Autodesk Inventor part; units mm, degrees
ref_plane "YZ Plane" through (0, 0, 0) normal (1, 0, 0) x (0, 1, 0)
ref_plane "XZ Plane" through (0, 0, 0) normal (0, 1, 0) x (-1, 0, 0)
ref_plane "XY Plane" through (0, 0, 0) normal (0, 0, 1) x (1, 0, 0)
sketch "Sketch1" plane through (0, 0, 0) normal (0, 1, 0) x (-1, 0, 0)
  line L0 (-104, 150) -> (104, 150)
  line L1 (150, 104) -> (150, -104)
  line L2 (104, -150) -> (-104, -150)
  line L3 (-150, -104) -> (-150, 104)
  line L4 (-150, 150) -> (150, -150) construction
  line L5 (150, 150) -> (-150, -150) construction
  line L6 (-100, 100) -> (100, 100) construction
  line L7 (100, 100) -> (100, -100) construction
  line L8 (100, -100) -> (-100, -100) construction
  line L9 (-100, -100) -> (-100, 100) construction
  line L10 (-100, 100) -> (100, -100) construction
  line L11 (100, 100) -> (-100, -100) construction
  line L12 (-125, 125) -> (125, 125) construction
  line L13 (125, 125) -> (125, -125) construction
  line L14 (125, -125) -> (-125, -125) construction
  line L15 (-125, -125) -> (-125, 125) construction
  line L16 (-125, 125) -> (125, -125) construction
  line L17 (125, 125) -> (-125, -125) construction
  line L18 (-75, 75) -> (75, 75) construction
  line L19 (75, 75) -> (75, -75) construction
  line L20 (75, -75) -> (-75, -75) construction
  line L21 (-75, -75) -> (-75, 75) construction
  line L22 (-75, 75) -> (75, -75) construction
  line L23 (75, 75) -> (-75, -75) construction
  line L24 (-104, -104) -> (104, -104) construction
  line L25 (104, -104) -> (104, 104) construction
  line L26 (104, 104) -> (-104, 104) construction
  line L27 (-104, 104) -> (-104, -104) construction
  circle A0 centre (125, -125) radius 1.5
  circle A1 centre (75, -75) radius 1.5
  circle A2 centre (75, 75) radius 1.5
  circle A3 centre (125, 125) radius 1.5
  circle A4 centre (-75, 75) radius 1.5
  circle A5 centre (-125, 125) radius 1.5
  circle A6 centre (-75, -75) radius 1.5
  circle A7 centre (-125, -125) radius 1.5
  line L28 (17.5, -100) -> (-17.5, -100)
  line L29 (-17.5, -100) -> (-17.5, -104)
  line L30 (-17.5, -104) -> (17.5, -104)
  line L31 (17.5, -104) -> (17.5, -100)
  arc A8 (104, -150) -> (150, -104) centre (104, -104) ccw
  arc A9 (150, 104) -> (104, 150) centre (104, 104) ccw
  arc A10 (-150, -104) -> (-104, -150) centre (-104, -104) ccw
  arc A11 (-104, 150) -> (-150, 104) centre (-104, 104) ccw
  line L32 (87.5, -100) -> (52.5, -100)
  line L33 (52.5, -100) -> (52.5, -104)
  line L34 (52.5, -104) -> (87.5, -104)
  line L35 (87.5, -104) -> (87.5, -100)
  line L36 (-87.5, -100) -> (-52.5, -100)
  line L37 (-52.5, -100) -> (-52.5, -104)
  line L38 (-52.5, -104) -> (-87.5, -104)
  line L39 (-87.5, -104) -> (-87.5, -100)
  line L40 (52.5, -104) -> (17.5, -100) construction
  line L41 (-17.5, -100) -> (-52.5, -104) construction
  line L42 (100, 17.5) -> (100, -17.5)
  line L43 (104, -17.5) -> (104, 17.5)
  line L44 (104, 17.5) -> (100, 17.5)
  line L45 (100, 52.5) -> (104, 52.5)
  line L46 (100, 87.5) -> (100, 52.5)
  line L47 (104, 87.5) -> (100, 87.5)
  line L48 (104, 52.5) -> (104, 87.5)
  line L49 (104, 52.5) -> (100, 17.5) construction
  line L50 (100, -17.5) -> (104, -17.5)
  line L51 (100, -17.5) -> (104, -52.5) construction
  line L52 (100, -52.5) -> (104, -52.5)
  line L53 (104, -87.5) -> (100, -87.5)
  line L54 (104, -52.5) -> (104, -87.5)
  line L55 (100, -87.5) -> (100, -52.5)
  line L56 (-17.5, 100) -> (17.5, 100)
  line L57 (17.5, 104) -> (-17.5, 104)
  line L58 (-17.5, 104) -> (-17.5, 100)
  line L59 (-52.5, 100) -> (-52.5, 104)
  line L60 (-87.5, 100) -> (-52.5, 100)
  line L61 (-87.5, 104) -> (-87.5, 100)
  line L62 (-52.5, 104) -> (-87.5, 104)
  line L63 (-52.5, 104) -> (-17.5, 100) construction
  line L64 (17.5, 100) -> (17.5, 104)
  line L65 (17.5, 100) -> (52.5, 104) construction
  line L66 (52.5, 100) -> (52.5, 104)
  line L67 (87.5, 104) -> (87.5, 100)
  line L68 (52.5, 104) -> (87.5, 104)
  line L69 (87.5, 100) -> (52.5, 100)
  line L70 (-100, -17.5) -> (-100, 17.5)
  line L71 (-104, 17.5) -> (-104, -17.5)
  line L72 (-104, -17.5) -> (-100, -17.5)
  line L73 (-100, -52.5) -> (-104, -52.5)
  line L74 (-100, -87.5) -> (-100, -52.5)
  line L75 (-104, -87.5) -> (-100, -87.5)
  line L76 (-104, -52.5) -> (-104, -87.5)
  line L77 (-104, -52.5) -> (-100, -17.5) construction
  line L78 (-100, 17.5) -> (-104, 17.5)
  line L79 (-100, 17.5) -> (-104, 52.5) construction
  line L80 (-100, 52.5) -> (-104, 52.5)
  line L81 (-104, 87.5) -> (-100, 87.5)
  line L82 (-104, 52.5) -> (-104, 87.5)
  line L83 (-100, 87.5) -> (-100, 52.5)
  point P0 (0, 0)
  point P1 (0, -100)
  point P2 (87.5, -102)
  point P3 (100, 0)
  point P4 (102, 87.5)
  point P5 (0, 100)
  point P6 (-87.5, 102)
  point P7 (-100, 0)
  point P8 (-102, -87.5)
  dimension "d0" = 300
  dimension "d1" = 300
  dimension "d2" = 200
  dimension "d3" = 200
  dimension "d4" = 4
  dimension "d5" = 25
  dimension "d6" = 25
  dimension "d7" = 3
  dimension "d8" = 3
  dimension "d11" = 360
  dimension "d16" = 4
  dimension "d24" = 46
  dimension "d25" = 46
  dimension "d31" = 35
  dimension "d32" = 35
  dimension "d35" = 360
extrude "Extrusion1" add sketch "Sketch1" along normal blind 4
sketch "Sketch3" plane through (0, 0, 0) normal (0, -1, 0) x (1, 0, 0)
  circle A0 centre (-35, 102) radius 1.5
  circle A1 centre (35, 102) radius 1.5
  line L0 (-52.5, 104) -> (-17.5, 100) construction
  line L1 (17.5, 100) -> (52.5, 104) construction
  circle A2 centre (-102, -35) radius 1.5
  circle A3 centre (-102, 35) radius 1.5
  circle A4 centre (35, -102) radius 1.5
  circle A5 centre (-35, -102) radius 1.5
  circle A6 centre (102, 35) radius 1.5
  circle A7 centre (102, -35) radius 1.5
  point P0 (0, 0)
  dimension "d44" = 3
  dimension "d45" = 3
  dimension "d48" = 360
extrude "Extrusion2" cut sketch "Sketch3" against normal up to next
sketch "Sketch4" plane through (0, 0, 0) normal (0, -1, 0) x (1, 0, 0)
  line L0 (87.5, -100) -> (-87.5, -100)
  line L1 (-87.5, -100) -> (-87.5, -104)
  line L2 (-87.5, -104) -> (-75, -104)
  line L3 (-75, -104) -> (-75, -135)
  line L4 (-75, -135) -> (75, -135)
  line L5 (75, -135) -> (75, -104)
  line L6 (75, -104) -> (87.5, -104)
  line L7 (87.5, -104) -> (87.5, -100)
  circle A0 centre (102, 35) radius 1.5
  circle A1 centre (-102, -35) radius 1.5
  circle A2 centre (-35, 102) radius 1.5
  circle A3 centre (102, -35) radius 1.5
  circle A4 centre (-102, 35) radius 1.5
  circle A5 centre (35, 102) radius 1.5
  circle A6 centre (125, -125) radius 1.5
  circle A7 centre (125, 125) radius 1.5
  circle A8 centre (-125, 125) radius 1.5
  circle A9 centre (-125, -125) radius 1.5
  line L8 (100, 17.5) -> (100, -17.5)
  line L9 (100, -17.5) -> (104, -17.5)
  line L10 (104, -17.5) -> (104, 17.5)
  line L11 (104, 17.5) -> (100, 17.5)
  line L12 (100, 52.5) -> (104, 52.5)
  line L13 (104, 52.5) -> (104, 87.5)
  line L14 (104, 87.5) -> (100, 87.5)
  line L15 (100, 87.5) -> (100, 52.5)
  line L16 (100, -52.5) -> (100, -87.5)
  line L17 (100, -87.5) -> (104, -87.5)
  line L18 (104, -87.5) -> (104, -52.5)
  line L19 (104, -52.5) -> (100, -52.5)
  line L20 (-17.5, 100) -> (17.5, 100)
  line L21 (17.5, 100) -> (17.5, 104)
  line L22 (17.5, 104) -> (-17.5, 104)
  line L23 (-17.5, 104) -> (-17.5, 100)
  line L24 (-52.5, 100) -> (-52.5, 104)
  line L25 (-52.5, 104) -> (-87.5, 104)
  line L26 (-87.5, 104) -> (-87.5, 100)
  line L27 (-87.5, 100) -> (-52.5, 100)
  line L28 (52.5, 100) -> (87.5, 100)
  line L29 (87.5, 100) -> (87.5, 104)
  line L30 (87.5, 104) -> (52.5, 104)
  line L31 (52.5, 104) -> (52.5, 100)
  line L32 (-100, -17.5) -> (-100, 17.5)
  line L33 (-100, 17.5) -> (-104, 17.5)
  line L34 (-104, 17.5) -> (-104, -17.5)
  line L35 (-104, -17.5) -> (-100, -17.5)
  line L36 (-100, -52.5) -> (-104, -52.5)
  line L37 (-104, -52.5) -> (-104, -87.5)
  line L38 (-104, -87.5) -> (-100, -87.5)
  line L39 (-100, -87.5) -> (-100, -52.5)
  line L40 (-100, 52.5) -> (-100, 87.5)
  line L41 (-100, 87.5) -> (-104, 87.5)
  line L42 (-104, 87.5) -> (-104, 52.5)
  line L43 (-104, 52.5) -> (-100, 52.5)
  circle A10 centre (-75, -75) radius 1.5
  circle A11 centre (-75, 75) radius 1.5
  circle A12 centre (75, 75) radius 1.5
  circle A13 centre (75, -75) radius 1.5
  arc A14 (-150, -104) -> (-104, -150) centre (-104, -104) ccw
  line L44 (-150, -104) -> (-150, 104)
  arc A15 (-104, 150) -> (-150, 104) centre (-104, 104) ccw
  line L45 (-104, 150) -> (104, 150)
  arc A16 (150, 104) -> (104, 150) centre (104, 104) ccw
  line L46 (150, 104) -> (150, -104)
  arc A17 (104, -150) -> (150, -104) centre (104, -104) ccw
  line L47 (104, -150) -> (-104, -150)
  circle A18 centre (-102, 35) radius 1.5
  circle A19 centre (102, -35) radius 1.5
  circle A20 centre (35, -102) radius 1.5
  circle A21 centre (35, 102) radius 1.5
  circle A22 centre (-102, -35) radius 1.5
  circle A23 centre (102, 35) radius 1.5
  circle A24 centre (-35, -102) radius 1.5
  circle A25 centre (-35, 102) radius 1.5
  circle A26 centre (-125, -125) radius 1.5
  circle A27 centre (-125, 125) radius 1.5
  circle A28 centre (125, 125) radius 1.5
  circle A29 centre (125, -125) radius 1.5
  line L48 (17.5, -100) -> (-17.5, -100)
  line L49 (-17.5, -100) -> (-17.5, -104)
  line L50 (-17.5, -104) -> (17.5, -104)
  line L51 (17.5, -104) -> (17.5, -100)
  line L52 (-52.5, -100) -> (-87.5, -100)
  line L53 (-87.5, -100) -> (-87.5, -104)
  line L54 (-87.5, -104) -> (-52.5, -104)
  line L55 (-52.5, -104) -> (-52.5, -100)
  line L56 (87.5, -104) -> (87.5, -100)
  line L57 (87.5, -100) -> (52.5, -100)
  line L58 (52.5, -100) -> (52.5, -104)
  line L59 (52.5, -104) -> (87.5, -104)
  line L60 (-100, -17.5) -> (-100, 17.5)
  line L61 (-100, 17.5) -> (-104, 17.5)
  line L62 (-104, 17.5) -> (-104, -17.5)
  line L63 (-104, -17.5) -> (-100, -17.5)
  line L64 (-104, 52.5) -> (-100, 52.5)
  line L65 (-100, 52.5) -> (-100, 87.5)
  line L66 (-100, 87.5) -> (-104, 87.5)
  line L67 (-104, 87.5) -> (-104, 52.5)
  line L68 (-100, -87.5) -> (-100, -52.5)
  line L69 (-100, -52.5) -> (-104, -52.5)
  line L70 (-104, -52.5) -> (-104, -87.5)
  line L71 (-104, -87.5) -> (-100, -87.5)
  line L72 (-17.5, 100) -> (17.5, 100)
  line L73 (17.5, 100) -> (17.5, 104)
  line L74 (17.5, 104) -> (-17.5, 104)
  line L75 (-17.5, 104) -> (-17.5, 100)
  line L76 (52.5, 104) -> (52.5, 100)
  line L77 (52.5, 100) -> (87.5, 100)
  line L78 (87.5, 100) -> (87.5, 104)
  line L79 (87.5, 104) -> (52.5, 104)
  line L80 (-87.5, 100) -> (-52.5, 100)
  line L81 (-52.5, 100) -> (-52.5, 104)
  line L82 (-52.5, 104) -> (-87.5, 104)
  line L83 (-87.5, 104) -> (-87.5, 100)
  line L84 (100, 17.5) -> (100, -17.5)
  line L85 (100, -17.5) -> (104, -17.5)
  line L86 (104, -17.5) -> (104, 17.5)
  line L87 (104, 17.5) -> (100, 17.5)
  line L88 (104, -52.5) -> (100, -52.5)
  line L89 (100, -52.5) -> (100, -87.5)
  line L90 (100, -87.5) -> (104, -87.5)
  line L91 (104, -87.5) -> (104, -52.5)
  line L92 (100, 87.5) -> (100, 52.5)
  line L93 (100, 52.5) -> (104, 52.5)
  line L94 (104, 52.5) -> (104, 87.5)
  line L95 (104, 87.5) -> (100, 87.5)
  circle A30 centre (75, -75) radius 1.5
  circle A31 centre (75, 75) radius 1.5
  circle A32 centre (-75, 75) radius 1.5
  circle A33 centre (-75, -75) radius 1.5
  arc A34 (104, -150) -> (150, -104) centre (104, -104) ccw
  line L96 (104, -150) -> (-104, -150)
  arc A35 (-150, -104) -> (-104, -150) centre (-104, -104) ccw
  line L97 (-150, -104) -> (-150, 104)
  arc A36 (-104, 150) -> (-150, 104) centre (-104, 104) ccw
  line L98 (-104, 150) -> (104, 150)
  arc A37 (150, 104) -> (104, 150) centre (104, 104) ccw
  line L99 (150, 104) -> (150, -104)
  line L100 (-75, -104) -> (-75, -100)
  line L101 (75, -104) -> (75, -100)
  point P0 (0, 0)
extrude "Extrusion3" add sketch "Sketch4" against normal up to surface (4 mm away) contours L101 L59 L58 L0 | L51 L50 L49 L0 | L55 L54 L100 L0 | A20 | A24
properties part number "Baseplate" material "MDF Medium Density Fiberboard"
Could you check a few things on this model? Use its own coordinates, in mm. Coordinates: 2 decimals unless noted, no trailing zeros. Order: outer loops, then holes, each group sorted by start corner. A loop starts at its lowest first (then second) coordinate and runs counter-clockwise, first axis right, second up. Notation, with made-up numbers: M 23.5,86 L 36.5,86 A35 ccw 36.5,123 Z; hole C 26,-29.75 d9. An arc over 180 degrees is marked long. Use one line per item in the form item = value. Start each with the question number.
1. Suppose I cut it at A-A on z = 84. Write out the boundary of the cut face in (x, y).
2. Please list where these lines run through material, in increasing order: line 1 (X direction, y = 2.4, z = 75); line 2 (X direction, y = 2.9, z = 81.5); line 3 (Z direction, x = -102, y = 2.35).
3. Suppose I cut it at B-B on y = 3.4. Count the separate pieces of the cut face and the enclosed holes in it, then the cut area to 3 significant figures.
4. For pin 1 (5 mm diameter, centred on x = -35, z = 102, fed in from -Y), with a flat end and sliding along its axis, tell me the tip position at first contact or that it passes through.
Geometry says:
q1.outline = M -150,0 L -104,0 L -104,4 L -150,4 Z; M -100,0 L 100,0 L 100,4 L -100,4 Z; M 104,0 L 150,0 L 150,4 L 104,4 Z
q2.line_1 = -150 to -104, -100 to -76.5, -73.5 to 73.5, 76.5 to 100, 104 to 150
q2.line_2 = -150 to -104, -100 to 100, 104 to 150
q2.line_3 = -150 to -87.5, -52.5 to -36.5, -33.5 to -17.5, 17.5 to 33.5, 36.5 to 52.5, 87.5 to 150
q3.separate_pieces = 1
q3.enclosed_holes = 25
q3.area = 86,700 mm^2
q4.pin_1 = 0
